CAD build for the part. Positions are in the model's coordinates, mm. Give positions to 0.01 mm unless a question says otherwise; leave off trailing zeros. Write each loop counter-clockwise with the first axis right and the second up, starting at its lowest first coordinate (ties: lowest second). Pieces come first, ordered by that corner, then holes. Notation, with made-up numbers: (23.25, 78.5) - (81.25, 78.5) arc R11 cw to (81.25, 84.5) - close; hole circle Ø3 at (-25.75, -29). An arc over 180 degrees is marked (long way). Answer as a JSON object with one key per item and string values.
from build123d import *

# Parameters (mm, degrees)
F0_W     = 19.05
F0_H     = 50.8
F1_DEPTH = 19.05


with BuildPart() as f1:
    # F0 (on Front) → F1 (new body)
    with BuildSketch(Plane.XZ):
        Polygon((-238.452145, -417.078608), (-238.452145, 27.421392), (-299.630938, 27.421392), (-423.838787, -436.128608), (-160.245545, -436.128608), (-160.245545, -455.178608), (-308.630615, -455.178608), (-308.630615, -474.228608), (-122.145545, -474.228608), (-122.145545, -417.078608), align=None)
        with Locations((-267.027145, -23.378608)):
            Rectangle(F0_W, F0_H, mode=Mode.SUBTRACT)
    extrude(amount=F1_DEPTH)


solid = f1.part
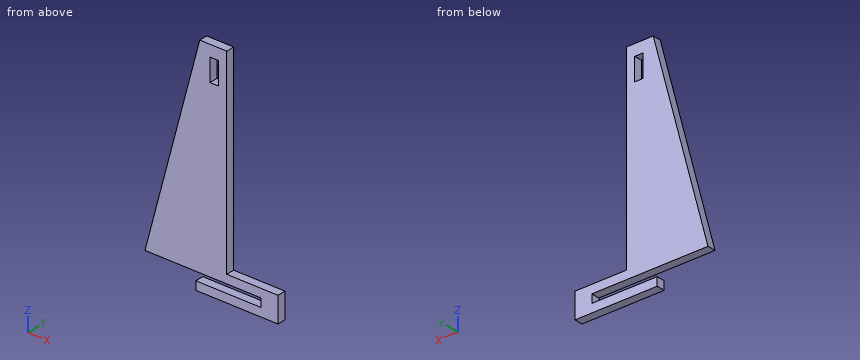
(1) Flat gauge pins, fed straight in: P1, Ø8, axis at y = -5.5, z = -111.5, coming from the +X side; P2, Ø1.5, axis at y = -8, z = -184, coming from the -X side; P3, Ø5.5, axis at y = -6.5, z = -463.5, coming from the -X side. Where does each tip first touch, or does it go through?
Answer key:
{"P1": "stops at x = -238.45", "P2": "stops at x = -356.48", "P3": "stops at x = -308.63"}
(2) Probe L1, parallel to Z at x = -250.5, y = -16.25; L2, parallel to Z at x = -188.5, y = -15.5; L3, parallel to Z at x = -136, y = -2.25. List the from-to ranges inside material, lowest first. Write a range as [from, to].
Answer key:
{"L1": "z = [-474.23, -455.18], [-436.13, 27.42]", "L2": "z = [-474.23, -455.18], [-436.13, -417.08]", "L3": "z = [-474.23, -417.08]"}
(3) Saw through at D-D, the plane x = -148. Give the cut face in (y, z), and give its area (3 significant figures).
Answer key:
{"outline": "(-19.05, -474.23) - (0, -474.23) - (0, -417.08) - (-19.05, -417.08) - close", "area": "1,090 mm²"}
(4) Saw through at A-A, the plane x = -187.5. Give the cut face in (y, z), and give its area (3 significant figures).
Answer key:
{"outline": "(-19.05, -474.23) - (0, -474.23) - (0, -455.18) - (-19.05, -455.18) - close; (-19.05, -436.13) - (0, -436.13) - (0, -417.08) - (-19.05, -417.08) - close", "area": "726 mm²"}
(5) Saw through at B-B, the plane y = -11.25. Give the cut face in (x, z).
Answer key:
{"outline": "(-423.84, -436.13) - (-160.25, -436.13) - (-160.25, -455.18) - (-308.63, -455.18) - (-308.63, -474.23) - (-122.15, -474.23) - (-122.15, -417.08) - (-238.45, -417.08) - (-238.45, 27.42) - (-299.63, 27.42) - close; hole (-276.55, -48.78) - (-257.5, -48.78) - (-257.5, 2.02) - (-276.55, 2.02) - close"}
(6) Saw through at C-C, the plane x = -266.5. Give the cut face in (y, z), and give its area (3 significant figures).
Answer key:
{"outline": "(-19.05, -474.23) - (0, -474.23) - (0, -455.18) - (-19.05, -455.18) - close; (-19.05, -436.13) - (0, -436.13) - (0, -48.78) - (-19.05, -48.78) - close; (-19.05, 2.02) - (0, 2.02) - (0, 27.42) - (-19.05, 27.42) - close", "area": "8,230 mm²"}
